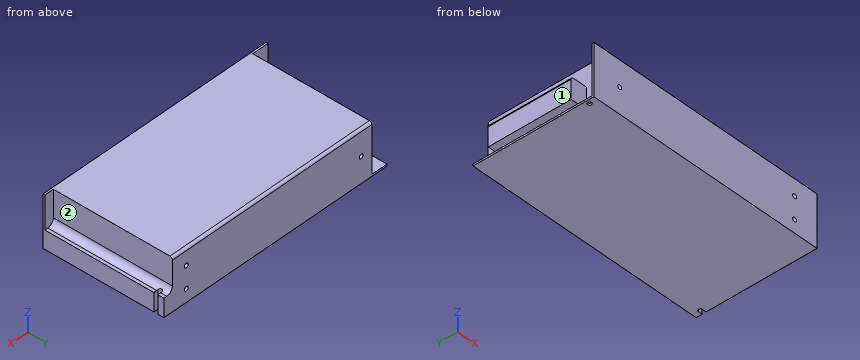
from build123d import *

# Parameters (mm, degrees)
F1_W      = 199
F1_H      = 42
F1_R      = 1.75
F2_DEPTH  = 99
F4_W      = 97.5
F4_H      = 27
F5_DEPTH  = 7.6
F6_R      = 5
F8_W      = 97.5
F8_H      = 40.5
F9_DEPTH  = 13.6
F10_W     = 68
F10_H     = 17.5
F11_DEPTH = 13.6
F12_R     = 2
F13_R     = 2
F15_R     = 1.6
F16_DEPTH = 42.001


# Not quite as in the source:
# - the program builds the solid bodies; features that only make, move or delete a surface that nothing else refers to are left out


with BuildPart() as f2:
    # F1 (on Front) → F2 (new body)
    with BuildSketch(Plane.XZ):
        Rectangle(F1_W, F1_H)
        with Locations((79.5, -10.5)):
            Circle(F1_R, mode=Mode.SUBTRACT)
        with Locations((-76.5, 0)):
            Circle(F1_R, mode=Mode.SUBTRACT)
        with Locations((79.5, 7.5)):
            Circle(F1_R, mode=Mode.SUBTRACT)
    extrude(amount=-F2_DEPTH)

    # F4 (on offset) → F5 (cut)
    with BuildSketch(Plane.YZ.offset(99.5)):
        with Locations((50.25, 7.5)):
            Rectangle(F4_W, F4_H)
    extrude(amount=-F5_DEPTH, mode=Mode.SUBTRACT)

    # F6
    f6_edges = [f2.edges().sort_by_distance(p)[0] for p in [
        (91.9, 50.25, -6),
    ]]
    fillet(f6_edges, radius=F6_R)

    # F8 (on offset) → F9 (cut)
    with BuildSketch(Plane(origin=(-99.5, 0, 0), x_dir=(0, -1, 0), z_dir=(-1, 0, 0))):
        with Locations((-50.25, 0.75)):
            Rectangle(F8_W, F8_H)
    extrude(amount=-F9_DEPTH, mode=Mode.SUBTRACT)

    # F10 (on offset) → F11 (join, through all)
    with BuildSketch(Plane(origin=(-99.5, 0, 0), x_dir=(0, -1, 0), z_dir=(-1, 0, 0))):
        with Locations((-52.6, -4.25)):
            Rectangle(F10_W, F10_H)
    extrude(amount=-F11_DEPTH)

    # F12
    f12_edges = [f2.edges().sort_by_distance(p)[0] for p in [
        (-99.5, 52.6, 4.5),
    ]]
    fillet(f12_edges, radius=F12_R)

    # F13
    f13_edges = [f2.edges().sort_by_distance(p)[0] for p in [
        (3, 99, 21),
    ]]
    fillet(f13_edges, radius=F13_R)

    # F15 (on face) → F16 (cut, through all)
    with BuildSketch(Plane(origin=(0, 0, -21), x_dir=(1, 0, 0), z_dir=(0, 0, -1))):
        with Locations((-96.3, -6.4)):
            Circle(F15_R)
        with BuildLine():
            Line((96, -94), (99.5, -94))
            Line((99.5, -94), (99.5, -90.8))
            Line((99.5, -90.8), (96, -90.8))
            ThreePointArc((96, -90.8), (97.1313708499, -91.2686291501), (97.6, -92.4))
            ThreePointArc((97.6, -92.4), (97.1313708499, -93.5313708499), (96, -94))
        make_face()
        with BuildLine():
            Line((96, -90.8), (96, -94))
            ThreePointArc((96, -94), (97.1313708499, -93.5313708499), (97.6, -92.4))
            ThreePointArc((97.6, -92.4), (97.1313708499, -91.2686291501), (96, -90.8))
        make_face()
        with BuildLine():
            ThreePointArc((96, -90.8), (94.4, -92.4), (96, -94))
            Line((96, -94), (96, -90.8))
        make_face()
    extrude(amount=-F16_DEPTH, mode=Mode.SUBTRACT)


solid = f2.part
Part model, mm, in its own coordinate system. Face numbers are marked on the shaded views. A direction names the side the tool comes from. Coordinates: 2 decimals unless noted, no trailing zeros. Order: outer loops, then holes, each group sorted by start corner. A loop starts at its lowest first (then second) coordinate and runs counter-clockwise, first axis right, second up. Notation, with made-up numbers: M 22,16.25 L 54,16.25 A17 cw 54,31.25 Z; hole C 8.25,9.25 d7. An arc over 180 degrees is marked long. One line per question, with ' | ' between items.
Q1. Slice it at C-C (y = 21). Give the cut face in (x, z).
A:
outline: M -99.5,-21 L 99.5,-21 L 99.5,-6 L 96.9,-6 A5 cw 91.9,-1 L 91.9,21 L -85.9,21 L -85.9,4.5 L -97.5,4.5 A2 ccw -99.5,2.5 L -99.5,-13 L -85.9,-13 L -85.9,-19.5 L -99.5,-19.5 Z; hole C -76.5,0 d3.5; hole C 79.5,-10.5 d3.5; hole C 79.5,7.5 d3.5
Q2. Slice it at D-D (z = -16). Give the cut face in (x, y), and give its area (3 significant figures).
A:
outline: M -99.5,0 L 99.5,0 L 99.5,90.8 L 96,90.8 A1.6 cw 96,94 L 99.5,94 L 99.5,99 L -85.9,99 L -85.9,1.5 L -99.5,1.5 Z | area: 18,400 mm^2
Q3. Drill centre lines: line 1 (Z direction, x = 79.5, y = 61); line 2 (Z direction, x = -90, y = 54); line 3 (X direction, y = 6.4, z = -20.55). Where is each one in solid material? Low to high.
A:
line 1: z = -21 to -12.25, -8.75 to 5.75, 9.25 to 21 | line 2: z = -21 to -19.5, -13 to 4.5 | line 3: x = -99.5 to -97.9, -94.7 to 99.5
Q4. Slice it at B-B (z = 15). Give the cut face in (x, y).
A:
outline: M -99.5,0 L 99.5,0 L 99.5,1.5 L 91.9,1.5 L 91.9,99 L -85.9,99 L -85.9,1.5 L -99.5,1.5 Z
Q5. 3-axis set-ups, long thin cutter, end or side, ignore diameter. For the marked faces 1 and 2: which of +Z, -Z, +X, -X, +Y, -Y reach the whole face in a straight line?
A:
face 1: +Z, -Z, -X, +Y, -Y | face 2: +Z, +X, +Y
Q6. Slice it at A-A (y = 88.5). Give the cut face in (x, z), and give its area (3 significant figures).
A:
outline: M -99.5,-21 L 99.5,-21 L 99.5,-6 L 96.9,-6 A5 cw 91.9,-1 L 91.9,21 L -85.9,21 L -85.9,-19.5 L -99.5,-19.5 Z; hole C -76.5,0 d3.5; hole C 79.5,-10.5 d3.5; hole C 79.5,7.5 d3.5 | area: 7,580 mm^2
Q7. Pin check, flat tips, straight feed: P1, Ø2, axis at x = 98.5, y = 96.5, coming from the +Z side; P2, Ø9.5, axis at x = -94.5, y = 43, coming from the +Z side; P3, Ø12, axis at y = 64.5, z = 13.5, coming from the +X side; P4, Ø2, axis at x = 79.5, z = -10.5, coming from the +Y side. Stop position of each tip, or through.
A:
P1: stops at z = -6 | P2: stops at z = 4.5 | P3: stops at x = 91.9 | P4: passes through
